Input: part model. Units: mm. Frame: model coordinates. Face numbers are marked on the shaded views. A direction names the side the tool comes from. Give positions to 0.01 mm unless a question says otherwise; leave off trailing zeros. Loops run counter-clockwise (first coordinate to the right, second up) from the corner with the lowest first, then second, coordinate; pieces in that order, holes last. Notation, with made-up numbers: (-26.5, 40.25) - (30.5, 40.25) arc R27 ccw to (30.5, 78.25) - close; hole circle Ø3 at (67.5, 25.5). An arc over 180 degrees is marked (long way). One line per item, written item: value.
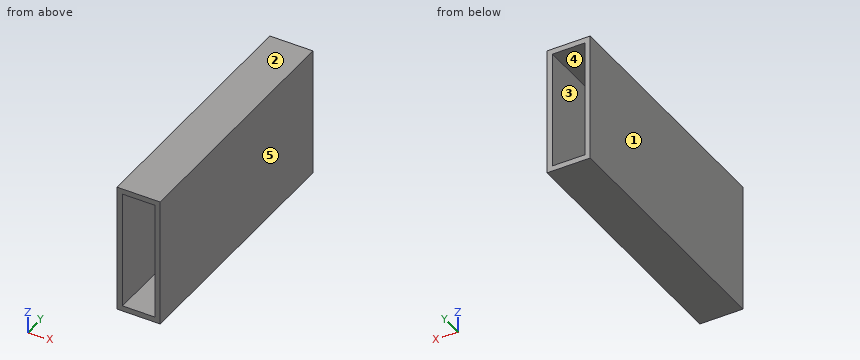
Autodesk Inventor part; units mm, degrees
ref_plane "YZ Plane" through (0, 0, 0) normal (1, 0, 0) x (0, 1, 0)
ref_plane "XZ Plane" through (0, 0, 0) normal (0, 1, 0) x (-1, 0, 0)
ref_plane "XY Plane" through (0, 0, 0) normal (0, 0, 1) x (1, 0, 0)
sketch "Sketch1" plane through (0, 0, 0) normal (0, 1, 0) x (-1, 0, 0)
  line L0 (-12.7, 76.2) -> (12.7, 76.2)
  line L1 (12.7, 76.2) -> (12.7, 0)
  line L2 (12.7, 0) -> (-12.7, 0)
  line L3 (-12.7, 0) -> (-12.7, 76.2)
  line L4 (9.525, 73.025) -> (-9.525, 73.025)
  line L5 (-9.525, 73.025) -> (-9.525, 3.175)
  line L6 (-9.525, 3.175) -> (9.525, 3.175)
  line L7 (9.525, 3.175) -> (9.525, 73.025)
  point P0 (0, 0)
  dimension "d0" = 25.4
  dimension "d1" = 76.2
  dimension "d2" = 0
  dimension "d3" = 12.7
  dimension "d4" = 3.175
extrude "Extrusion1" add sketch "Sketch1" along normal mid plane 152.4
properties part number "2x4 StandIn- 2021"
Item 1: Pin query (flat end, axial travel): P1, Ø10, axis at x = 2.5, z = 64, coming from the -Y side. Return the tip coordinate at first contact, or that it passes through.
Verdict:
P1: passes through
Item 2: Material intervals for L1, parallel to X at y = 27, z = 68 (3 decimals); L2, parallel to Z at x = -9.25, y = 46.5 (3 decimals), sorted ascending.
Verdict:
L1: x = -12.7 to -9.525, 9.525 to 12.7
L2: z = 0 to 3.175, 73.025 to 76.2
Item 3: Section A-A, the plane x = -1.75. Output: boundary loops of the cut face in (y, z) (3 decimals).
Verdict:
outline: (-76.2, 0) - (76.2, 0) - (76.2, 3.175) - (-76.2, 3.175) - close; (-76.2, 73.025) - (76.2, 73.025) - (76.2, 76.2) - (-76.2, 76.2) - close
Item 4: Access query for the marked faces 4 and 5. Directions: +Z, -Z, +X, -X, +Y, -Y. A direction counts if a zero-diameter tool reaches every point of the face in a straight line with its end or side. Return the directions, or none.
Verdict:
face 4: +Y, -Y
face 5: +Z, -Z, +X, +Y, -Y
Item 5: Section C-C, the plane z = 62. Output: boundary loops of the cut face in (x, y) (3 decimals), and give its area (3 significant figures).
Verdict:
outline: (-12.7, -76.2) - (-9.525, -76.2) - (-9.525, 76.2) - (-12.7, 76.2) - close; (9.525, -76.2) - (12.7, -76.2) - (12.7, 76.2) - (9.525, 76.2) - close
area: 968 mm^2
Item 6: Draft query along Z for the marked faces 1, 2 and 3. Return one class per face: pulls with the +Z half, pulls with the -Z half, needs draft (parallel to the pull), parting line crosses it, or undercut.
Verdict:
face 1: needs draft
face 2: pulls with the +Z half
face 3: undercut
Item 7: Section B-B, the plane y = -50. Output: boundary loops of the cut face in (x, z) (3 decimals).
Verdict:
outline: (-12.7, 0) - (12.7, 0) - (12.7, 76.2) - (-12.7, 76.2) - close; hole (-9.525, 3.175) - (9.525, 3.175) - (9.525, 73.025) - (-9.525, 73.025) - close
